```python
from build123d import *

# Parameters (mm, degrees)
MODEL_R             = 8.1
MODEL_R_2           = 1.5
MODEL_R_3           = 2.525
MODEL_R_4           = 15
BOSS_EXTRUDE1_DEPTH = 4


with BuildPart() as part:
    # Model → Boss-Extrude1 (new body)
    with BuildSketch(Plane.XY):
        with BuildLine():
            Line((-93.5, -16), (-73.5, -16))
            Line((-73.5, -16), (-73.5, -36))
            ThreePointArc((-73.5, -36), (-70.571067812, -43.071067812), (-63.5, -46))
            Line((-63.5, -46), (-43.5, -46))
            Line((-43.5, -46), (-43.5, -66))
            Line((-43.5, -66), (43.5, -66))
            Line((43.5, -66), (43.5, -46))
            Line((43.5, -46), (63.5, -46))
            ThreePointArc((63.5, -46), (70.571067812, -43.071067812), (73.5, -36))
            Line((73.5, -36), (73.5, -16))
            Line((73.5, -16), (93.5, -16))
            Line((93.5, -16), (93.5, 16))
            Line((93.5, 16), (73.5, 16))
            Line((73.5, 16), (73.5, 36))
            ThreePointArc((73.5, 36), (70.571067812, 43.071067812), (63.5, 46))
            Line((63.5, 46), (43.5, 46))
            Line((43.5, 46), (43.5, 86))
            Line((43.5, 86), (-43.5, 86))
            Line((-43.5, 86), (-43.5, 46))
            Line((-43.5, 46), (-63.5, 46))
            ThreePointArc((-63.5, 46), (-70.571067812, 43.071067812), (-73.5, 36))
            Line((-73.5, 36), (-73.5, 16))
            Line((-73.5, 16), (-93.5, 16))
            Line((-93.5, 16), (-93.5, -16))
        make_face()
        with Locations((23.5, 31)):
            Circle(MODEL_R, mode=Mode.SUBTRACT)
        with Locations((-26.5, 31)):
            Circle(MODEL_R_2, mode=Mode.SUBTRACT)
        with Locations((-58.5, 31)):
            Circle(MODEL_R_2, mode=Mode.SUBTRACT)
        with Locations((83.5, 0)):
            Circle(MODEL_R_3, mode=Mode.SUBTRACT)
        with Locations((0, 76)):
            Circle(MODEL_R_3, mode=Mode.SUBTRACT)
        with Locations((-83.5, 0)):
            Circle(MODEL_R_3, mode=Mode.SUBTRACT)
        with Locations((0, -56)):
            Circle(MODEL_R_3, mode=Mode.SUBTRACT)
        with Locations((-58.5, -1)):
            Circle(MODEL_R_2, mode=Mode.SUBTRACT)
        with Locations((58.5, 31)):
            Circle(MODEL_R, mode=Mode.SUBTRACT)
        with Locations((-42.5, 15)):
            Circle(MODEL_R_4, mode=Mode.SUBTRACT)
        with BuildLine():
            Line((58.5, -1), (-26.5, -1))
            ThreePointArc((-26.5, -1), (-30.035533906, -2.464466094), (-31.5, -6))
            Line((-31.5, -6), (-31.5, -26))
            ThreePointArc((-31.5, -26), (-30.035533906, -29.535533906), (-26.5, -31))
            Line((-26.5, -31), (58.5, -31))
            ThreePointArc((58.5, -31), (62.035533906, -29.535533906), (63.5, -26))
            Line((63.5, -26), (63.5, -6))
            ThreePointArc((63.5, -6), (62.035533906, -2.464466094), (58.5, -1))
        make_face(mode=Mode.SUBTRACT)
    extrude(amount=BOSS_EXTRUDE1_DEPTH)


solid = part.part
```
The model under review builds one solid part; all positions refer to its coordinate system, in mm. A direction names the side the tool comes from. Round coordinates to 2 decimals unless told otherwise and drop trailing zeros. Loops run counter-clockwise (first coordinate to the right, second up) from the corner with the lowest first, then second, coordinate; pieces in that order, holes last.
1) Consider section C-C on z = 2.85. Give the number of separate pieces and of enclosed holes in the cut face, then the cut area to 3 significant figures.
Values follow:
separate pieces: 1
enclosed holes: 11
area: 15,900 mm2
2) Wall thickness on line 1 along Y through (x, z) = (23.5, 2.55); line 2 along X through (y, z) = (-15.5, 0.7); line 3 along Y through (x, z) = (-10, 2): over which ranges is each line inside the solid? List them lowest first.
Values follow:
line 1: y = -66 to -31, -1 to 22.9, 39.1 to 86
line 2: x = -93.5 to -31.5, 63.5 to 93.5
line 3: y = -66 to -31, -1 to 86
3) Consider section D-D on y = 58.5. State the section outline as (x, z) points.
Values follow:
outline: (-43.5, 0) - (43.5, 0) - (43.5, 4) - (-43.5, 4) - close
4) Consider section B-B on y = 11. State the section outline as (x, z) points.
Values follow:
outline: (-93.5, 0) - (-56.96, 0) - (-56.96, 4) - (-93.5, 4) - close; (-28.04, 0) - (93.5, 0) - (93.5, 4) - (-28.04, 4) - close
5) Consider section A-A on x = 39. State the section outline as (y, z) points.
Values follow:
outline: (-66, 0) - (-31, 0) - (-31, 4) - (-66, 4) - close; (-1, 0) - (86, 0) - (86, 4) - (-1, 4) - close
6) Tool access review of faces 1 (the face through (53, -46, 2)), 2 (the face through (-31.5, -16, 2)), 3 (the face through (-53, 46, 2)): name each direction out of +Z, -Z, +X, -X, +Y, -Y from which nothing blocks a thin tool from reaching the whole face with its end or side.
Values follow:
face 1: +Z, -Z, +X, -Y
face 2: +Z, -Z
face 3: +Z, -Z, -X, +Y
7) The part is to be moulded in two halves that separate along Y. For faces 4 (the face through (17, -1, 2)), 5 (the face through (70.65, 42.99, 1.97)), 6 (the face through (-43.5, 66, 2)), say which applies: pulls with the +Y half, pulls with the -Y half, needs draft (parallel to the pull), parting line crosses it, or undercut.
Values follow:
face 4: undercut
face 5: pulls with the +Y half
face 6: needs draft
8) Clearance check with flat-ended pins moving along their axes: P1, Ø1.2, axis at x = 49.5, z = 2.5, coming from the -Y side; P2, Ø2, axis at y = -54.5, z = 3, coming from the +X side; P3, Ø3, axis at x = 0, y = 76, coming from the -Z side; P4, Ø1.5, axis at y = -50.5, z = 2.5, coming from the -X side. State where each tip first meets the part, or that it passes through.
Values follow:
P1: stops at y = -46
P2: stops at x = 43.5
P3: passes through
P4: stops at x = -43.5
